Geometry: final body of the model. Coordinates: model frame, mm. Face numbers are marked on the shaded views. A direction names the side the tool comes from. Give positions to 0.01 mm unless a question says otherwise; leave off trailing zeros. Write each loop counter-clockwise with the first axis right and the second up, starting at its lowest first coordinate (ties: lowest second). Pieces come first, ordered by that corner, then holes. Notation, with made-up numbers: (21, 19.5) -> (73, 19.5) arc R21 cw to (73, 23.5) -> close; hole circle Ø8 at (-17.5, 37.5). An arc over 180 degrees is marked (long way). Answer as a JSON object with one key per item and string values. Group by question number.
(1) Section query D-D on y = 20.5. Output: boundary loops of the cut face in (x, z), plus the area to 3 significant figures.
(2) Section query A-A on x = -43. Output: boundary loops of the cut face in (y, z), plus the area to 3 significant figures.
(3) Draft query along X for the marked faces 1, 2 and 3. Return one class per face: +X half, -X half, draft (parallel to the pull), parting line (faces both ways), or undercut.
(4) Contact query for flat-ended pins moving along their axis: pin 1 Ø20 at (y, z) = (26, 19) entering from +X; pin 2 Ø2 at (x, y) = (-52, 5.5) entering from -Z; pin 3 Ø10 at (x, z) = (-66, 32.5) entering from -Y; pin 4 Ø3.5 at (y, z) = (2, 3) entering from -X. Output: stop coordinate, or through.
(5) Material intervals for probe 1 along Z at (x, y) = (-18, 2.5); probe 2 along X at (y, z) = (12, 40.5); probe 3 along Y at (x, z) = (-37, 40), sorted ascending.
(6) Section query B-B on y = 9. Output: boundary loops of the cut face in (x, z), plus the area to 3 significant figures.
(7) Section query C-C on z = 36.5. Output: boundary loops of the cut face in (x, y).
(8) Set-up query: the marked faces 4 and 5. Return all of +Z, -Z, +X, -X, +Y, -Y with unobstructed straight access to the full face (end or side cutting, diameter ignored); none if empty.
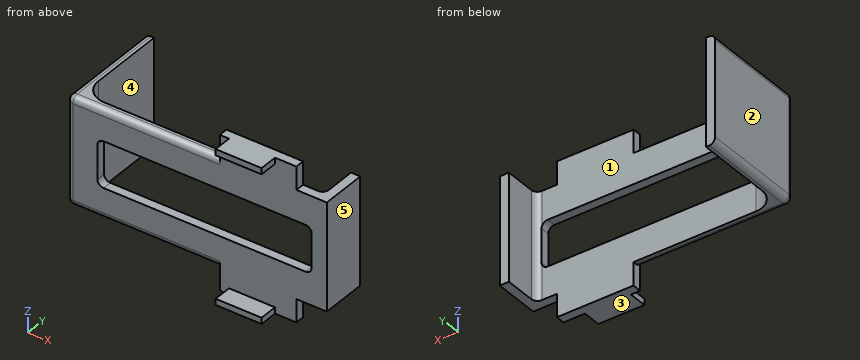
Autodesk Inventor part; units mm, degrees
ref_plane "YZ Plane" through (0, 0, 0) normal (1, 0, 0) x (0, 1, 0)
ref_plane "XZ Plane" through (0, 0, 0) normal (0, 1, 0) x (-1, 0, 0)
ref_plane "XY Plane" through (0, 0, 0) normal (0, 0, 1) x (1, 0, 0)
sketch "Skizze1" plane through (0, 0, 0) normal (0, 1, 0) x (-1, 0, 0)
  line L0 (0, 0) -> (25, 0)
  line L1 (25, 50) -> (0, 50)
  line L2 (0, 42.5) -> (-9.9167, 42.5)
  line L3 (-9.9167, 42.5) -> (-9.9167, 7.5)
  line L4 (-9.9167, 7.5) -> (0, 7.5)
  line L5 (65, 32.5) -> (-5, 32.5)
  line L6 (-5, 32.5) -> (-5, 17.5)
  line L7 (-5, 17.5) -> (65, 17.5)
  line L8 (65, 17.5) -> (65, 32.5)
  line L9 (0, 7.5) -> (0, 17.5)
  line L10 (0, 32.5) -> (0, 42.5)
  line L11 (0, 50) -> (0, 32.5)
  line L12 (0, 17.5) -> (0, 0)
  line L13 (25, 42.5) -> (75, 42.5)
  line L14 (75, 42.5) -> (75, 7.5)
  line L15 (75, 7.5) -> (25, 7.5)
  line L16 (25, 0) -> (25, 17.5)
  line L17 (25, 32.5) -> (25, 50)
  dimension "d0" = 50
  dimension "d1" = 25
  dimension "d2" = 7.5
  dimension "d4" = 35
  dimension "d5" = 10
  dimension "d6" = 15
  dimension "d8" = 70
  dimension "d9" = 65
  dimension "d26" = 50
  dimension "d27" = 35
  dimension "d28" = 7.5
extrude "Extrusion1" add sketch "Skizze1" along normal blind 3 contours L12 L9 L7 L16 L0 | L4 L3 L2 L10 L5 L6 L7 L9 | L16 L7 L8 L5 L17 L13 L14 L15 | L11 L1 L17 L5 L10
sketch "Skizze2" plane through (0, 0, 42.5) normal (0, 0, 1) x (1, 0, 0)
  line L0 (9.9167, 0) -> (9.9167, 3)
  line L1 (9.9167, 3) -> (6.9167, 3)
  line L2 (6.9167, 3) -> (6.9167, 15)
  line L3 (6.9167, 15) -> (9.9167, 15)
  line L4 (9.9167, 15) -> (9.9167, 3)
  point P0 (0, 0)
  dimension "d12" = 3
  dimension "d13" = 12
extrude "Extrusion2" add sketch "Skizze2" against normal up to surface (35 mm away)
fillet "Rundung1" radius 2 1 edges at (6.9167, 3, 25)
sketch "Skizze3" plane through (0, 0, 0) normal (0, -1, 0) x (1, 0, 0)
  line L0 (-22, 0) -> (-7, 0)
  line L1 (-7, 0) -> (-7, 2)
  line L2 (-7, 2) -> (-22, 2)
  line L3 (-22, 2) -> (-22, 0)
  line L4 (-22, 48) -> (-7, 48)
  line L5 (-7, 48) -> (-7, 50)
  line L6 (-7, 50) -> (-22, 50)
  line L7 (-22, 50) -> (-22, 48)
  line L8 (-25, 50) -> (0, 50)
  line L9 (0, 50) -> (0, 42.5)
  point P0 (0, 0)
  point P1 (0, 32.5)
  dimension "d17" = 2
  dimension "d18" = 2
  dimension "d19" = 46
  dimension "d20" = 15
  dimension "d21" = 15
  dimension "d22" = 0
  dimension "d23" = 7
extrude "Extrusion3" add sketch "Skizze3" along normal blind 6
sketch "Skizze4" plane through (-75, 0, 7.5) normal (-1, 0, 0) x (0, 0, 1)
  line L0 (0, 0) -> (0, 35)
  line L1 (0, 35) -> (35, 35)
  line L2 (35, 0) -> (35, 15)
  line L3 (35, 35) -> (35, 0)
  line L4 (0, 0) -> (0, 15)
  line L5 (35, 0) -> (0, 0)
  point P0 (-7.5, 0)
  dimension "d29" = 35
extrude "Extrusion4" add sketch "Skizze4" against normal blind 3
fillet "Rundung2" radius 7 1 edges at (-72, 3, 25)
fillet "Rundung3" radius 2 7 edges at (-50, 0, 42.5) (-75, 0, 25) (-50, 0, 7.5) (-65, 1.5, 17.5) (-65, 1.5, 32.5) (5, 1.5009, 32.5) (5, 1.5009, 17.5)
fillet "Rundung4" radius 2 4 edges at (-74.4142, 0.5858, 41.9142) (-75, 18.5, 42.5) (-74.4142, 0.5858, 8.0858) (-75, 18.5, 7.5)
properties part number "Ultrasonic" material "Stahl, Guss"
Answer list:
{
 "1": {"outline": "(-75, 9.5) arc R2 ccw to (-73, 7.5) -> (-72, 7.5) -> (-72, 42.5) -> (-73, 42.5) arc R2 ccw to (-75, 40.5) -> close", "area": "103 mm2"},
 "2": {"outline": "(0, 9.5) arc R2 ccw to (2, 7.5) -> (3, 7.5) -> (3, 17.5) -> (0, 17.5) -> close; (0, 32.5) -> (3, 32.5) -> (3, 42.5) -> (2, 42.5) arc R2 ccw to (0, 40.5) -> close", "area": "58.3 mm2"},
 "3": {"face 1": "undercut", "face 2": "-X half", "face 3": "draft"},
 "4": {"pin 1": "x = -72", "pin 2": "through", "pin 3": "y = 0", "pin 4": "x = -25"},
 "5": {"probe 1": "0 to 17.5, 32.5 to 50", "probe 2": "-75 to -72, 6.92 to 9.92", "probe 3": "0 to 3"},
 "6": {"outline": "(-75, 9.5) arc R2 ccw to (-73, 7.5) -> (-71.93, 7.5) -> (-71.93, 42.5) -> (-73, 42.5) arc R2 ccw to (-75, 40.5) -> close; (6.92, 7.5) -> (9.92, 7.5) -> (9.92, 42.5) -> (6.92, 42.5) -> close", "area": "211 mm2"},
 "7": {"outline": "(-75, 2) arc R2 ccw to (-73, 0) -> (9.92, 0) -> (9.92, 15) -> (6.92, 15) -> (6.92, 5) arc R2 cw to (4.92, 3) -> (-65, 3) arc R7 cw to (-72, 10) -> (-72, 35) -> (-75, 35) -> close"},
 "8": {"face 4": "+Z, -Z, +Y", "face 5": "+Z, -Z, +X, +Y, -Y"}
}
